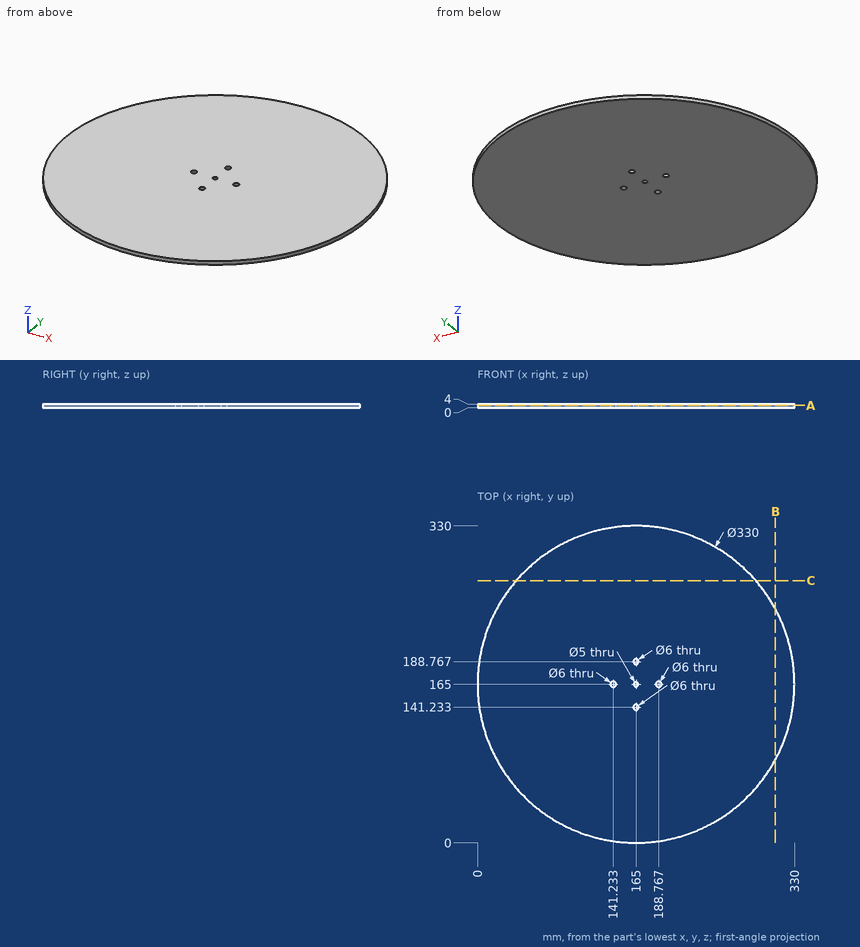
Print and shaded views of the part. All mm, measured from the part's lowest x, y and z. Give positions to 0.01 mm unless a question says otherwise; leave off trailing zeros. Write each loop counter-clockwise with the first axis right and the second up, starting at its lowest first coordinate (ties: lowest second). Pieces come first, ordered by that corner, then holes. Notation, with made-up numbers: M 15.25,41 L 25.25,41 A11 cw 25.25,62 Z; hole C 59,-25 d6. An arc over 180 degrees is marked long. Use a Markdown table: item, result.
1) Pin check, flat tips, straight feed: pin 1 (2 mm diameter, centred on y = 281, z = 1, fed in from +X); pin 2 (2 mm diameter, centred on y = 112, z = 1, fed in from -X). Stop position of each tip, or through.
Responses:
| item | result |
|---|---|
| pin 1 | stops at x = 283.32 |
| pin 2 | stops at x = 8.41 |
2) Drill centre lines: line 1 (Y direction, x = 165, z = 1.5); line 2 (Y direction, x = 312.5, z = 2.7); line 3 (X direction, y = 176.5, z = 3.8). Where is each one in solid material? Low to high. Write a range as from..to.
Responses:
| item | result |
|---|---|
| line 1 | y = 0..138.23, 144.23..162.5, 167.5..185.77, 191.77..330 |
| line 2 | y = 91.05..238.95 |
| line 3 | x = 0.4..329.6 |
3) Cut at A-A (z = 2.65). List the corners of the cut face in (x, y).
Responses:
| item | result |
|---|---|
| outline | C 165,165 d330; hole C 141.23,165 d6; hole C 165,141.23 d6; hole C 165,188.77 d6; hole C 165,165 d5; hole C 188.77,165 d6 |
4) Cut at C-C (y = 273). List the corners of the cut face in (x, z), and give its area (3 significant figures).
Responses:
| item | result |
|---|---|
| outline | M 40.26,0 L 289.74,0 L 289.74,4 L 40.26,4 Z |
| area | 998 mm2 |
5) Cut at B-B (x = 310). List the corners of the cut face in (y, z).
Responses:
| item | result |
|---|---|
| outline | M 86.26,0 L 243.74,0 L 243.74,4 L 86.26,4 Z |
